Here's how the part is built. I have some questions about the finished solid (model axes, mm). A direction names the side the tool comes from. Coordinates: 2 decimals unless noted, no trailing zeros. Write each loop counter-clockwise with the first axis right and the second up, starting at its lowest first coordinate (ties: lowest second). Pieces come first, ordered by that corner, then holes. Notation, with made-up numbers: (8.5, 10.25) - (40.5, 10.25) arc R16 cw to (40.5, 22.25) - close; hole circle Ø1 at (-39.5, 56.5). An arc over 180 degrees is marked (long way). Answer in a Markdown table with one row per item. Add a question column.
Item 1: I'm going to push flat-ended pins straight in: pin 1 (12 mm diameter, centred on x = 25, z = 58.5, fed in from +Y); pin 2 (3 mm diameter, centred on y = -22.5, z = 181, fed in from +X); pin 3 (5 mm diameter, centred on x = -6, z = 38, fed in from -Y). Where does each tip first touch, or does it pass through?
Item 2: We'd pull the mould along Y, two halves only. Please class faces 1 (the face through (-39.329, -30.156, 125.785)), 2 (the face through (9, 16.5, 250)), 3 (the face through (19, -19, 6)): +Y half, -Y half, draft (parallel to the pull), parting line (faces both ways), or undercut.
Item 3: Imagine slicing it at A-A (y = 0). Please give me the cut outline in (x, z), plus the area to 3 significant figures.
Item 4: Which directions (+Z, -Z, +X, -X, +Y, -Y) give clear straight access to the entire face, cutting with the end or side of a thin tool? Please do faces 4 (the face through (11.32, -21.77, 126.29)), 5 (the face through (0, -44, 250)).
Item 5: If I drill on probe 1 along Y at (x, z) = (0, 135.5); probe 2 along Y at (x, z) = (-19.5, 204.5); probe 3 along X at (y, z) = (-11, 182.5), over which ranges is the centre line in solid material (lowest first)? Write a range as from..to.
Item 6: Imagine slicing it at B-B (z = 211). Please give me the cut outline in (x, y).
from build123d import *

# Parameters (mm, degrees)
F0_R     = 49.559661
F0_R_2   = 18.538097
F1_DEPTH = 250
F2_R     = 5
F3_T     = -6


with BuildPart() as f1:
    # F0 (on Top) → F1 (new body)
    with BuildSketch(Plane.XY):
        Circle(F0_R)
        Circle(F0_R_2, mode=Mode.SUBTRACT)
    extrude(amount=F1_DEPTH)

    # F2
    f2_edges = [f1.edges().sort_by_distance(p)[0] for p in [
        (-49.559661, 0, 0),
    ]]
    fillet(f2_edges, radius=F2_R)

    # F3
    f3_openings = [f1.faces().sort_by_distance(p)[0] for p in [
        (-48.157902, 0, 250),
    ]]
    offset(amount=F3_T, openings=f3_openings)


solid = f1.part
Here are the results:
| question | item | result |
|---|---|---|
| 1 | pin 1 | stops at y = 45.77 |
| 1 | pin 2 | stops at x = 44.89 |
| 1 | pin 3 | stops at y = -49.44 |
| 2 | face 1 | parting line |
| 2 | face 2 | draft |
| 2 | face 3 | undercut |
| 3 | outline | (-49.56, 5) arc R5 ccw to (-44.56, 0) - (-18.54, 0) - (-18.54, 250) - (-24.54, 250) - (-24.54, 6) - (-43.56, 6) - (-43.56, 250) - (-49.56, 250) - close; (18.54, 0) - (44.56, 0) arc R5 ccw to (49.56, 5) - (49.56, 250) - (43.56, 250) - (43.56, 6) - (24.54, 6) - (24.54, 250) - (18.54, 250) - close |
| 3 | area | 6,220 mm2 |
| 4 | face 4 | +Z |
| 4 | face 5 | +Z, +X, -X, +Y, -Y |
| 5 | probe 1 | y = -49.56..-43.56, -24.54..-18.54, 18.54..24.54, 43.56..49.56 |
| 5 | probe 2 | y = -45.56..-38.95, -14.9..14.9, 38.95..45.56 |
| 5 | probe 3 | x = -48.32..-42.15, -21.93..-14.92, 14.92..21.93, 42.15..48.32 |
| 6 | outline | circle Ø99.12 at (0, 0); circle Ø49.08 at (0, 0); hole circle Ø87.12 at (0, 0); hole circle Ø37.08 at (0, 0) |
